Could you check a few things on this drawing? It's one solid part, dimensions in mm from its lowest x, y, z. A direction names the side the tool comes from. Give positions to 0.01 mm unless a question says otherwise; leave off trailing zeros. Loops run counter-clockwise (first coordinate to the right, second up) from the corner with the lowest first, then second, coordinate; pieces in that order, holes last. Notation, with made-up numbers: M -20.75,31.5 L 35.25,31.5 A27 cw 35.25,53.5 Z; hole C -0.75,-11 d9. An arc over 180 degrees is marked long. Answer in a Markdown table with one row per item. Add a question column.
1. I need wall thicknesses on line 1 along Z through (x, y) = (19.5, 2.75); line 2 along Y through (x, z) = (13, 16); line 3 along Y through (x, z) = (9.5, 3). Which ranges of each line are inside material? Lowest first, please. Write a range as from..to.
2. Which directions (+Z, -Z, +X, -X, +Y, -Y) give clear straight access to the entire face, cutting with the end or side of a thin tool? Please do the marked faces 1 and 2.
3. If we section it at D-D on z = 28: List the corners of the cut face in (x, y) for me, then the cut area to 3 significant figures.
4. I'm going to push flat-ended pins straight in: pin 1 Ø2 at (x, z) = (25, 18) entering from +Y; pin 2 Ø2.5 at (x, y) = (10.5, 4.5) entering from -Z. Where does each tip first touch, or does it pass through?
5. If we section it at C-C on z = 10: List the corners of the cut face in (x, y) for me.
6. If we section it at B-B on x = 30.5: List the corners of the cut face in (y, z) for me, then the cut area to 3 significant figures.
7. If we section it at A-A on y = 3.45: List the corners of the cut face in (x, z) for me.
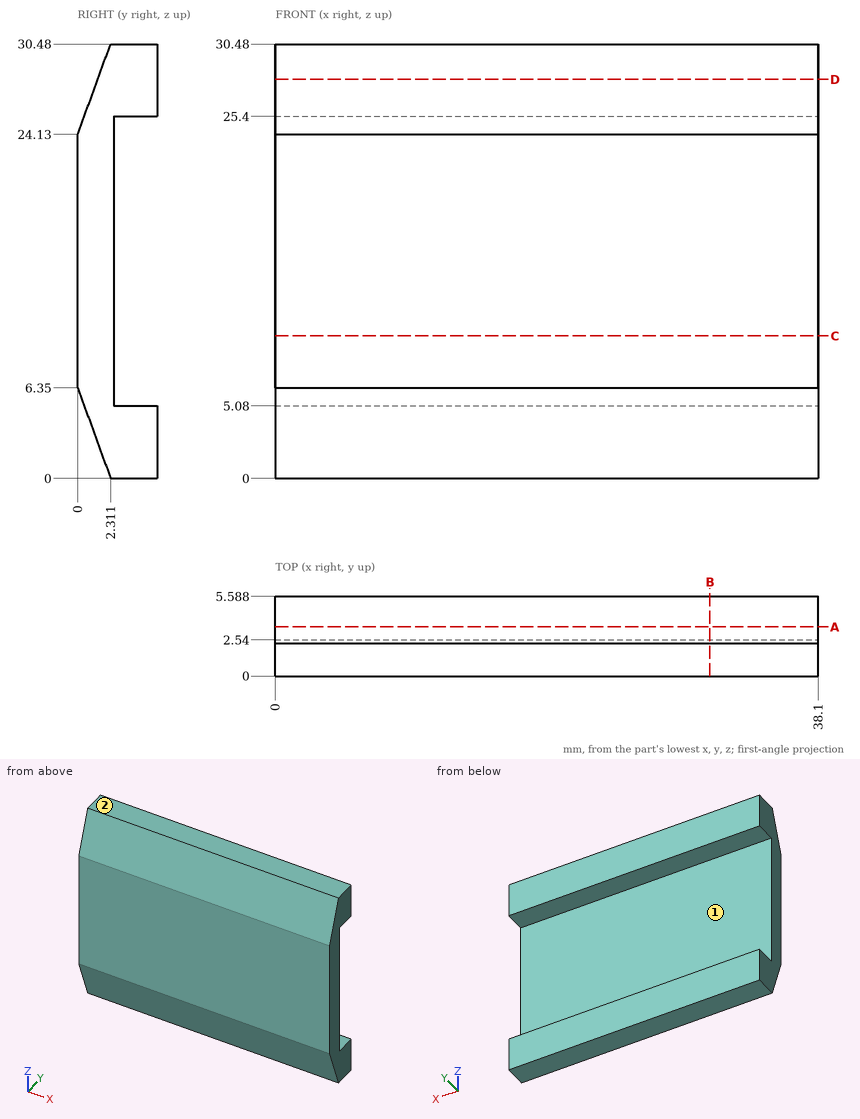
Results:
| question | item | result |
|---|---|---|
| 1 | line 1 | 0..5.08, 25.4..30.48 |
| 1 | line 2 | 0..2.54 |
| 1 | line 3 | 1.22..5.59 |
| 2 | face 1 | +X, -X, +Y |
| 2 | face 2 | +Z, +X, -X, +Y, -Y |
| 3 | outline | M 0,1.41 L 38.1,1.41 L 38.1,5.59 L 0,5.59 Z |
| 3 | area | 159 mm2 |
| 4 | pin 1 | y = 2.54 |
| 4 | pin 2 | z = 0 |
| 5 | outline | M 0,0 L 38.1,0 L 38.1,2.54 L 0,2.54 Z |
| 6 | outline | M 0,6.35 L 2.31,0 L 5.59,0 L 5.59,5.08 L 2.54,5.08 L 2.54,25.4 L 5.59,25.4 L 5.59,30.48 L 2.31,30.48 L 0,24.13 Z |
| 6 | area | 93.7 mm2 |
| 7 | outline | M 0,0 L 38.1,0 L 38.1,5.08 L 0,5.08 Z; M 0,25.4 L 38.1,25.4 L 38.1,30.48 L 0,30.48 Z |
